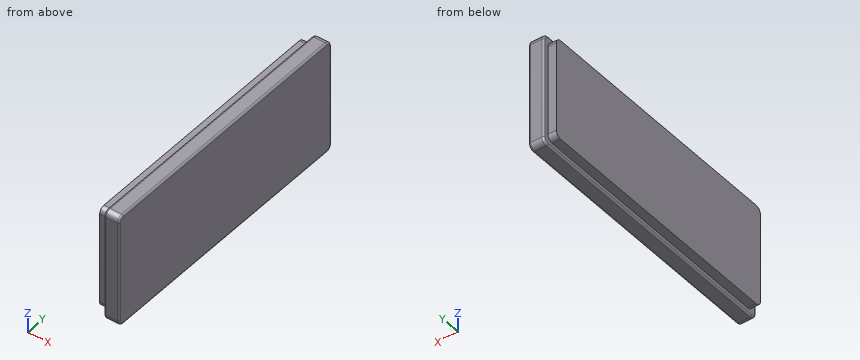
from build123d import *

# Parameters (mm, degrees)
PAD_DEPTH    = 4.5
PAD001_DEPTH = 8
FILLET_R     = 1


with BuildPart() as part:
    # Sketch → Pad (new body)
    with BuildSketch(Plane.YZ):
        with BuildLine():
            Line((-65, 27), (71, 27))
            ThreePointArc((74, 24), (73.12132, 26.12132), (71, 27))
            Line((74, 24), (74, -24))
            ThreePointArc((71, -27), (73.12132, -26.12132), (74, -24))
            Line((71, -27), (-65, -27))
            ThreePointArc((-68, -24), (-67.12132, -26.12132), (-65, -27))
            Line((-68, -24), (-68, 24))
            ThreePointArc((-65, 27), (-67.12132, 26.12132), (-68, 24))
        make_face()
    extrude(amount=-PAD_DEPTH)

    # Sketch001 → Pad001 (join)
    with BuildSketch(Plane.YZ):
        with BuildLine():
            Line((-67.828427, 29.828427), (73.828427, 29.828427))
            ThreePointArc((76.828427, 26.828427), (75.949747, 28.949747), (73.828427, 29.828427))
            Line((76.828427, 26.828427), (76.828427, -26.828427))
            ThreePointArc((73.828427, -29.828427), (75.949747, -28.949747), (76.828427, -26.828427))
            Line((73.828427, -29.828427), (-67.828427, -29.828427))
            ThreePointArc((-70.828427, -26.828427), (-69.949747, -28.949747), (-67.828427, -29.828427))
            Line((-70.828427, -26.828427), (-70.828427, 26.828427))
            ThreePointArc((-67.828427, 29.828427), (-69.949747, 28.949747), (-70.828427, 26.828427))
        make_face()
    extrude(amount=PAD001_DEPTH)

    # Fillet
    fillet_edges = [part.edges().sort_by_distance(p)[0] for p in [
        (0, 3, 29.828427),
        (0, -69.949747, 28.949747),
        (0, -70.828427, 0),
        (8, -69.949747, 28.949747),
        (8, -70.828427, 0),
        (8, 3, 29.828427),
        (0, -69.949747, -28.949747),
        (8, -69.949747, -28.949747),
        (8, 3, -29.828427),
        (0, 3, -29.828427),
        (0, 75.949747, -28.949747),
        (8, 75.949747, -28.949747),
        (0, 76.828427, 0),
        (8, 76.828427, 0),
        (0, 75.949747, 28.949747),
        (8, 75.949747, 28.949747),
    ]]
    fillet(fillet_edges, radius=FILLET_R)


solid = part.part
For this review, take the finished solid that the model builds, in its own axes (mm). Give positions to 0.01 mm unless a question says otherwise; leave off trailing zeros. Order: outer loops, then holes, each group sorted by start corner. A loop starts at its lowest first (then second) coordinate and runs counter-clockwise, first axis right, second up. Notation, with made-up numbers: (-33.75, 23) - (-14.75, 23) arc R22 ccw to (-14.75, 51) - close; hole circle Ø3 at (34, -19.75). An arc over 180 degrees is marked (long way). Answer as a JSON object with one key per item and string values. Group by question number.
Item 1: Take a section at A-A on x = -2.75. Give the boundary of the cut face in (y, z).
Item 2: Take a section at B-B on y = -50. Give the boundary of the cut face in (x, z).
Item 3: Wall thickness on line 1 along Y through (x, z) = (-0.5, -8.5); line 2 along Z through (x, y) = (-0.75, 43); line 3 along Y through (x, z) = (0.75, -17): over which ranges is each line inside the solid? List them lowest first.
Item 4: Clearance check with flat-ended pins moving along their axes: pin 1 Ø2 at (x, y) = (-1.5, 15) entering from +Z; pin 2 Ø1.3 at (x, y) = (-2.5, -19.5) entering from -Z; pin 3 Ø6 at (x, y) = (-2.5, -34) entering from -Z. State where each tip first meets the part, or that it passes through.
Reported:
{
 "1": {"outline": "(-68, -24) arc R3 ccw to (-65, -27) - (71, -27) arc R3 ccw to (74, -24) - (74, 24) arc R3 ccw to (71, 27) - (-65, 27) arc R3 ccw to (-68, 24) - close"},
 "2": {"outline": "(-4.5, -27) - (0, -27) - (0, -28.83) arc R1 ccw to (1, -29.83) - (7, -29.83) arc R1 ccw to (8, -28.83) - (8, 28.83) arc R1 ccw to (7, 29.83) - (1, 29.83) arc R1 ccw to (0, 28.83) - (0, 27) - (-4.5, 27) - close"},
 "3": {"line 1": "-68 to 74", "line 2": "-27 to 27", "line 3": "-70.8 to 76.8"},
 "4": {"pin 1": "z = 27", "pin 2": "z = -27", "pin 3": "z = -29.69"}
}
